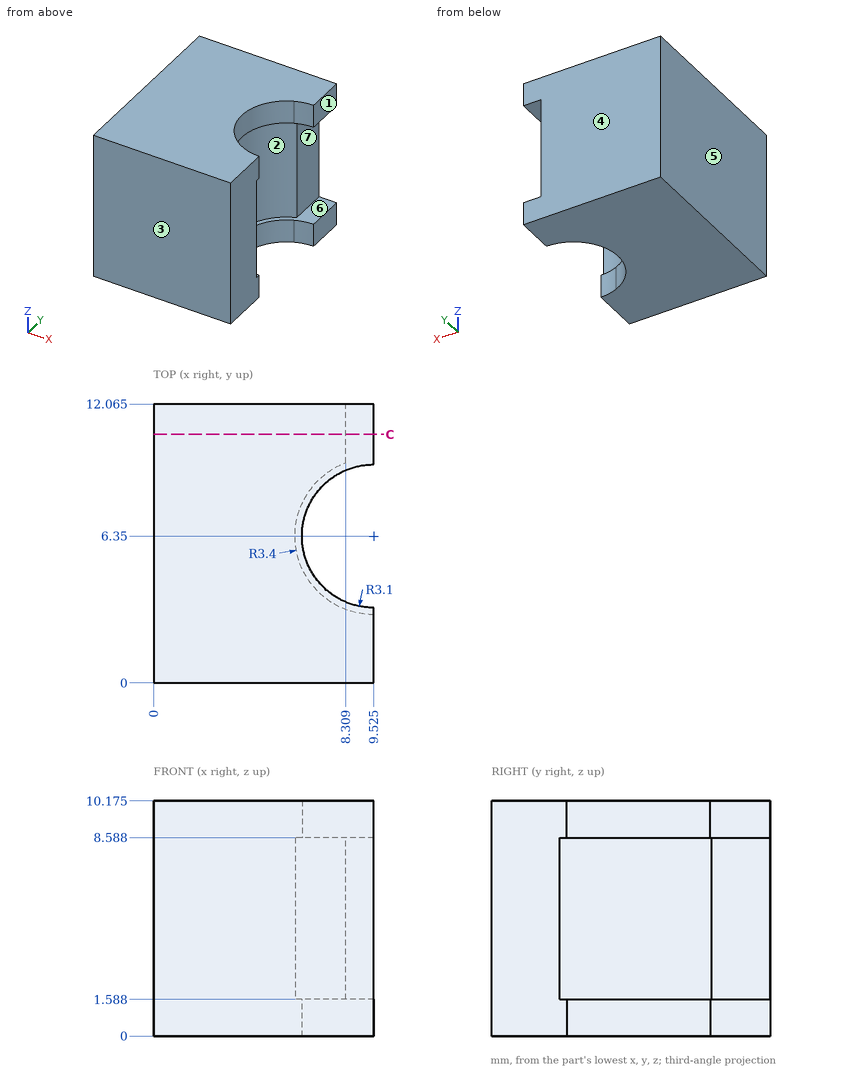
Print and shaded views of the part. All mm, measured from the part's lowest x, y and z. A direction names the side the tool comes from. Coordinates: 2 decimals unless noted, no trailing zeros. Order: outer loops, then holes, each group sorted by start corner. A loop starts at its lowest first (then second) coordinate and runs counter-clockwise, first axis right, second up. Notation, with made-up numbers: (-6, -39.75) -> (3, -39.75) arc R26 ccw to (3, -9.75) -> close; hole circle Ø6 at (49, 76). An arc over 180 degrees is marked (long way). Answer as a JSON object with one key per item and string values. Group by question number.
1) Which spindle directions (+Z, -Z, +X, -X, +Y, -Y) get a long thin tool onto all of the face, cutting with end or side? Do the marked faces 5, 6 and 7. Say none if no direction does.
2) Flat gauge pins, fed straight in: pin 1 (3.5 mm diameter, centred on x = 8, y = 7.5, fed in from -Z); pin 2 (0.8 mm diameter, centred on y = 10.5, z = 5, fed in from +X); pin 3 (3 mm diameter, centred on y = 6.5, z = 3.5, fed in from +X); pin 4 (2 mm diameter, centred on y = 5.5, z = 3.5, fed in from +X). Where does each tip first touch, or does it go through?
3) Pull direction Y, two halves, no side cores. Call the marked faces 1, 2, 3 and 4: +Y half, -Y half, draft (parallel to the pull), parting line (faces both ways), or undercut.
4) Drill centre lines: L1, parallel to Z at x = 7.75, y = 3.75 (1 decimal); L2, parallel to Y at x = 9, z = 0.75 (1 decimal); L3, parallel to Y at x = 6.75, z = 4 (1 decimal). Where is each one in solid material? Low to high.
5) Cut at C-C, the plane y = 10.75. Write the cut outline in (x, z) (1 decimal), then the cut area to 3 significant figures.
Check values:
{
 "1": {"face 5": "+Z, -Z, -X, +Y, -Y", "face 6": "+X", "face 7": "+X, +Y"},
 "2": {"pin 1": "stops at z = 0", "pin 2": "stops at x = 8.31", "pin 3": "stops at x = 6.55", "pin 4": "stops at x = 6.67"},
 "3": {"face 1": "draft", "face 2": "undercut", "face 3": "-Y half", "face 4": "+Y half"},
 "4": {"L1": "z = 0 to 1.6, 8.6 to 10.2", "L2": "y = 0 to 3.3, 9.4 to 12.1", "L3": "y = 0 to 4.4, 8.3 to 12.1"},
 "5": {"outline": "(0, 0) -> (9.5, 0) -> (9.5, 1.6) -> (8.3, 1.6) -> (8.3, 8.6) -> (9.5, 8.6) -> (9.5, 10.2) -> (0, 10.2) -> close", "area": "88.4 mm²"}
}
